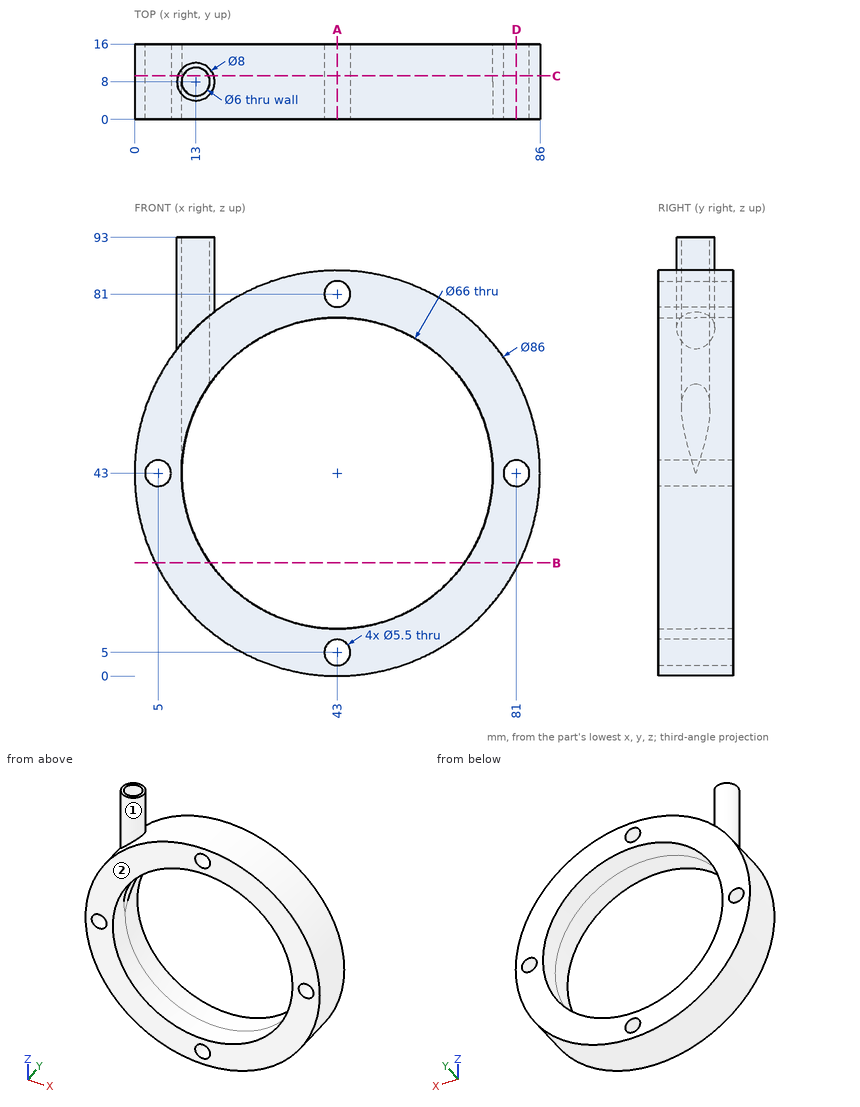
For this review, use the dimensioned drawing (mm, ordinates from the lowest corner) and the shaded views. A direction names the side the tool comes from. Round coordinates to 2 decimals unless told otherwise and drop trailing zeros. Loops run counter-clockwise (first coordinate to the right, second up) from the corner with the lowest first, then second, coordinate; pieces in that order, holes last. Notation, with made-up numbers: M 60,-29.5 L 81,-29.5 A28 ccw 81,-10.5 Z; hole C 65.25,5 d11. An arc over 180 degrees is marked long. Answer as a JSON object with one key per item and string values.
(1) Take a section at D-D on x = 81. Give the boundary of the cut face in (y, z).
Resolved:
{"outline": "M 0,22.88 L 16,22.88 L 16,40.25 L 0,40.25 Z; M 0,45.75 L 16,45.75 L 16,63.12 L 0,63.12 Z"}
(2) To check wall thickness, follow line 1 along X through (y, z) = (6.25, 42.5); line 2 along Y through (x, z) = (13, 79); line 3 along X through (y, z) = (3.75, 37.5). State the ranges of each line that lie inside material, in increasing order.
Resolved:
{"line 1": "0 to 2.3, 7.7 to 10, 76 to 78.3, 83.7 to 86", "line 2": "4 to 5, 11 to 12", "line 3": "0.35 to 10.46, 75.54 to 85.65"}
(3) Take a section at C-C on y = 9.25. Give the boundary of the cut face in (x, z), and give its area (3 significant figures).
Resolved:
{"outline": "M 9.2,69.58 A43 ccw long 16.8,77.1 L 16.8,93 L 15.73,93 L 15.73,61.58 A33 cw long 10.27,47.23 L 10.27,93 L 9.2,93 Z; hole C 5,43 d5.5; hole C 43,5 d5.5; hole C 43,81 d5.5; hole C 81,43 d5.5", "area": "2,240 mm²"}
(4) Take a section at B-B on z = 24. Give the boundary of the cut face in (x, y), and give its area (3 significant figures).
Resolved:
{"outline": "M 4.43,0 L 16.02,0 L 16.02,16 L 4.43,16 Z; M 69.98,0 L 81.57,0 L 81.57,16 L 69.98,16 Z", "area": "371 mm²"}
(5) Tool access review of the marked faces 1 and 2: name each direction out of +Z, -Z, +X, -X, +Y, -Y from which nothing blocks a thin tool from reaching the whole face with its end or side.
Resolved:
{"face 1": "+Z", "face 2": "+Z, -Z, +X, -X, -Y"}
(6) Take a section at A-A on x = 43. Give the boundary of the cut face in (y, z).
Resolved:
{"outline": "M 0,0 L 16,0 L 16,2.25 L 0,2.25 Z; M 0,7.75 L 16,7.75 L 16,10 L 0,10 Z; M 0,76 L 16,76 L 16,78.25 L 0,78.25 Z; M 0,83.75 L 16,83.75 L 16,86 L 0,86 Z"}
(7) Clearance check with flat-ended pins moving along their axes: P1, Ø1, axis at y = 14, z = 58, coming from the -X side; P2, Ø8, axis at x = 75.5, y = 5.5, coming from the +Z side; P3, Ø5, axis at x = 43, z = 81, coming from the -Y side; P4, Ø8, axis at x = 56, y = 12, coming from the -Z side. State where each tip first meets the part, or that it passes through.
Resolved:
{"P1": "x = 2.52", "P2": "z = 75.2", "P3": "through", "P4": "z = 0.95"}
